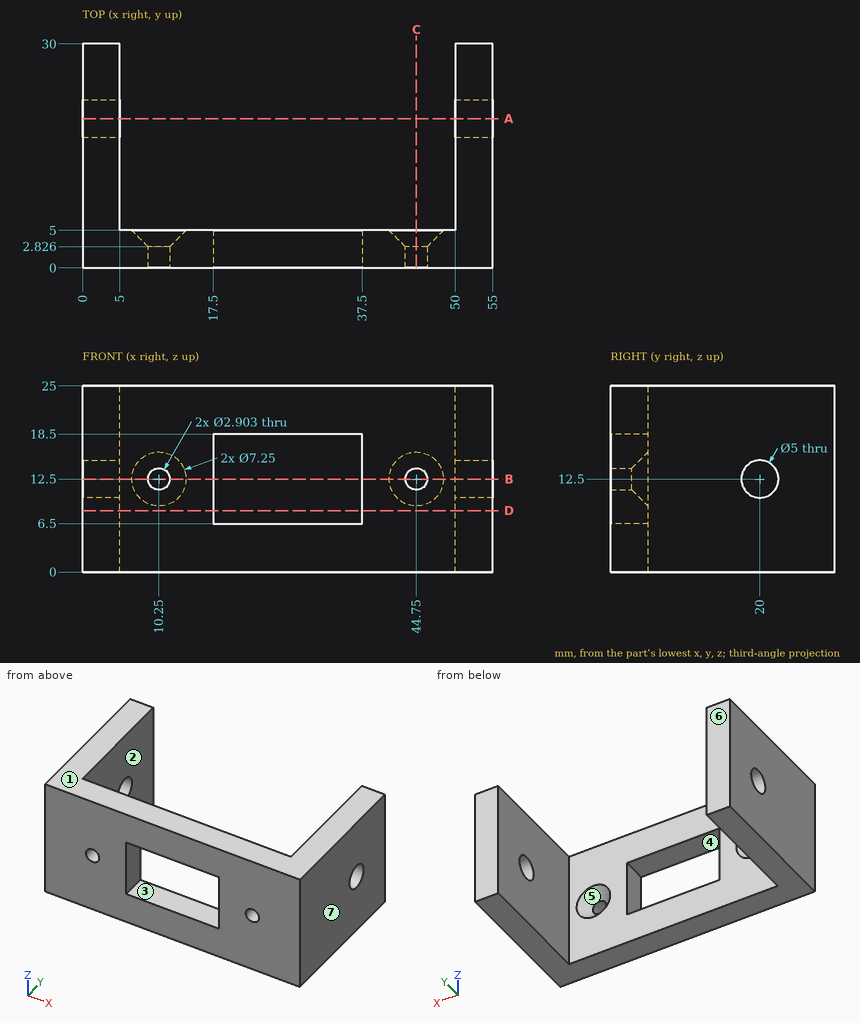
Answer from the drawing. Dimensions are ordinates in mm from the lowest x, y and z of the part. A direction names the side the tool comes from. Coordinates: 2 decimals unless noted, no trailing zeros. Order: outer loops, then holes, each group sorted by start corner. A loop starts at its lowest first (then second) coordinate and runs counter-clockwise, first axis right, second up. Notation, with made-up numbers: M 44,-26.5 L 78,-26.5 A18 cw 78,-14.5 Z; hole C 18.5,34 d1. An arc over 180 degrees is marked long. Put each result on its own line as item: value. Start each with the question number.
Item 1: Consider probe 1 along X at (y, z) = (1.1, 12.5); probe 2 along X at (y, z) = (22.25, 6.5); probe 3 along Y at (x, z) = (1.25, 12.5). Determine where each line is inside the solid, lowest interval first. Write a range as [from, to].
Item 2: Section A-A, the plane y = 20 is taken. Determine the outline of the cut face in (x, z).
Item 3: Given pin 1 Ø4 at (y, z) = (2.5, 13.5) entering from -X; pin 2 Ø6 at (x, z) = (40, 5.5) entering from +Y, each flat-ended and moving along its own axis, determine where each tip first touches the part or whether it passes through.
Item 4: Section C-C, the plane x = 44.75 is taken. Determine the outline of the cut face in (y, z) (1 decimal), plus the area to 3 significant figures.
Item 5: For the marked faces 1, 2 and 3, determine the directions among +Z, -Z, +X, -X, +Y, -Y from which every point of the face is accessible in a straight line to the end or side of a thin tool.
Item 6: Section D-D, the plane z = 8.25 is taken. Determine the outline of the cut face in (x, y), plus the area to 3 significant figures.
Item 7: Section B-B, the plane z = 12.5 is taken. Count the separate pieces of the cut face and the enclosed holes in it.
Item 8: The mould has two halves that part along X. Classify the marked faces 4, 5, 6 and 7: +X half, -X half, draft (parallel to the pull), parting line (faces both ways), or undercut.
Computed:
1. probe 1: x = [0, 8.8], [11.7, 17.5], [37.5, 43.3], [46.2, 55]
1. probe 2: x = [0, 5], [50, 55]
1. probe 3: y = [0, 17.5], [22.5, 30]
2. outline: M 0,0 L 5,0 L 5,10 L 0,10 Z; M 0,15 L 5,15 L 5,25 L 0,25 Z; M 50,0 L 55,0 L 55,10 L 50,10 Z; M 50,15 L 55,15 L 55,25 L 50,25 Z
3. pin 1: stops at x = 0
3. pin 2: stops at y = 5
4. outline: M 0,0 L 5,0 L 5,8.9 L 2.8,11 L 0,11 Z; M 0,14 L 2.8,14 L 5,16.1 L 5,25 L 0,25 Z
4. area: 106 mm2
5. face 1: +Z, +X, -X, +Y, -Y
5. face 2: +Z, -Z, +Y
5. face 3: +Y, -Y
6. outline: M 0,0 L 17.5,0 L 17.5,5 L 5,5 L 5,30 L 0,30 Z; M 37.5,0 L 55,0 L 55,30 L 50,30 L 50,5 L 37.5,5 Z
6. area: 425 mm2
7. separate pieces: 6
7. enclosed holes: 0
8. face 4: undercut
8. face 5: undercut
8. face 6: draft
8. face 7: +X half
